Geometry check sheet. Reference: the model listing, model coordinates, mm. Give positions to 0.01 mm unless a question says otherwise; leave off trailing zeros. Loops run counter-clockwise (first coordinate to the right, second up) from the corner with the lowest first, then second, coordinate; pieces in that order, holes last. Notation, with made-up numbers: (35.25, 28) -> (50.25, 28) arc R31 ccw to (50.25, 63) -> close; hole circle Ø10 at (13, -26.75). An arc over 180 degrees is marked (long way). Write item = value, one per line.
```python
from build123d import *

# Parameters (mm, degrees)
SKETCH072_W     = 452.6
SKETCH072_H     = 368
PAD026_DEPTH    = 12
SKETCH073_W     = 452.6
SKETCH073_H     = 6
POCKET044_DEPTH = 6
SKETCH074_W     = 452.6
SKETCH074_H     = 6
POCKET045_DEPTH = 6
SKETCH075_W     = 6
SKETCH075_H     = 356
POCKET046_DEPTH = 6


with BuildPart() as part:
    # Sketch072 → Pad026 (new body)
    with BuildSketch(Plane.XY):
        with Locations((0, 184)):
            Rectangle(SKETCH072_W, SKETCH072_H)
    extrude(amount=PAD026_DEPTH)

    # Sketch073 (on Face5 of Pad026) → Pocket044 (cut)
    with BuildSketch(Plane(origin=(0, 0, 0), x_dir=(1, 0, 0), z_dir=(0, 0, -1))):
        with Locations((0, -3)):
            Rectangle(SKETCH073_W, SKETCH073_H)
    extrude(amount=-POCKET044_DEPTH, mode=Mode.SUBTRACT)

    # Sketch074 (on Face4 of Pocket044) → Pocket045 (cut)
    with BuildSketch(Plane(origin=(0, 0, 0), x_dir=(1, 0, 0), z_dir=(0, 0, -1))):
        with Locations((0, -365)):
            Rectangle(SKETCH074_W, SKETCH074_H)
    extrude(amount=-POCKET045_DEPTH, mode=Mode.SUBTRACT)

    # Sketch075 (on Face7 of Pocket045) → Pocket046 (cut)
    with BuildSketch(Plane(origin=(0, 0, 0), x_dir=(1, 0, 0), z_dir=(0, 0, -1))):
        with Locations((-223.3, -184)):
            Rectangle(SKETCH075_W, SKETCH075_H)
    pocket046 = extrude(amount=-POCKET046_DEPTH, mode=Mode.SUBTRACT)

    # Mirrored017: Pocket046 across Sketch075 V_Axis
    add(pocket046.mirror(Plane(origin=(0, 0, 0), x_dir=(0, 0, -1), z_dir=(1, 0, 0))), mode=Mode.SUBTRACT)


with BuildPart() as part_1:
    # Body025 placement: moved
    add(part.part.moved(Location((0, -6, 0))))


solid = part_1.part
```
Item 1: Section check A-A, the plane x = -140.5. Record the cut outline in (y, z), plus the area to 3 significant figures.
Answer:
outline = (-6, 6) -> (0, 6) -> (0, 0) -> (356, 0) -> (356, 6) -> (362, 6) -> (362, 12) -> (-6, 12) -> close
area = 4,340 mm^2
Item 2: Thickness scan on L1, parallel to Y at x = 30, z = 4.25; L2, parallel to X at y = 126, z = 4.75. Record the ranges inside material, lowest first. Write a range as [from, to].
Answer:
L1 = [0, 356]
L2 = [-220.3, 220.3]
Item 3: Gauge pin test, flat ends, axial feed: pin 1 (3 mm diameter, centred on y = 132, z = 2, fed in from -X); pin 2 (3 mm diameter, centred on y = 181.5, z = 3, fed in from +X); pin 3 (1 mm diameter, centred on x = 138, z = 4, fed in from +Y). Record the tip position at first contact, or that the pin passes through.
Answer:
pin_1 = -220.3
pin_2 = 220.3
pin_3 = 356
Item 4: Section check B-B, the plane z = 3. Record the cut outline in (x, y).
Answer:
outline = (-220.3, 0) -> (220.3, 0) -> (220.3, 356) -> (-220.3, 356) -> close
